from build123d import *

# Parameters (mm, degrees)
SKETCH_1_W          = 280
SKETCH_1_H          = 274
EXTRUDE_1_DEPTH     = 18
SKETCH_2_W          = 520
SKETCH_2_H          = 10
EXTRUDE_2_DEPTH     = 172
CUT_EXTRUDE_1_DEPTH = 466.041933593
CUT_EXTRUDE_2_DEPTH = 466.041933593
SKETCH_5_R          = 11
CUT_EXTRUDE_3_DEPTH = 521.745619281
SKETCH_6_R          = 11
CUT_EXTRUDE_4_DEPTH = 521.745619281
SKETCH_7_R          = 11
CUT_EXTRUDE_5_DEPTH = 521.745619281
SKETCH_8_R          = 11
CUT_EXTRUDE_6_DEPTH = 521.745619281
SKETCH_9_R          = 11
CUT_EXTRUDE_8_DEPTH = 466.041933593


with BuildPart() as part:
    # 草图1 → 拉伸1 (new body)
    with BuildSketch(Plane.XY):
        with Locations((140, 137)):
            Rectangle(SKETCH_1_W, SKETCH_1_H)
    extrude(amount=EXTRUDE_1_DEPTH)

    # 草图2 → 拉伸2 (add)
    with BuildSketch(Plane.XY.offset(18)):
        with Locations((140, 137)):
            Rectangle(SKETCH_2_W, SKETCH_2_H)
    extrude(amount=EXTRUDE_2_DEPTH)

    # 草图3 → 切除-拉伸1 (cut, through all)
    with BuildSketch(Plane.XZ.offset(-132)):
        Polygon((0, 18), (-120, 115), (-120, 18), align=None)
    extrude(amount=-CUT_EXTRUDE_1_DEPTH, mode=Mode.SUBTRACT)

    # 草图4 → 切除-拉伸2 (cut, through all)
    with BuildSketch(Plane.XZ.offset(-132)):
        Polygon((400, 115), (280, 18), (400, 18), align=None)
    extrude(amount=-CUT_EXTRUDE_2_DEPTH, mode=Mode.SUBTRACT)

    # 草图5 → 切除-拉伸3 (cut, through all)
    with BuildSketch(Plane(origin=(0, 0, 0), x_dir=(-1, 0, 0), z_dir=(0, 0, -1))):
        with Locations((-210, 35)):
            Circle(SKETCH_5_R)
    extrude(amount=-CUT_EXTRUDE_3_DEPTH, mode=Mode.SUBTRACT)

    # 草图6 → 切除-拉伸4 (cut, through all)
    with BuildSketch(Plane(origin=(0, 0, 0), x_dir=(-1, 0, 0), z_dir=(0, 0, -1))):
        with Locations((-210, 239)):
            Circle(SKETCH_6_R)
    extrude(amount=-CUT_EXTRUDE_4_DEPTH, mode=Mode.SUBTRACT)

    # 草图7 → 切除-拉伸5 (cut, through all)
    with BuildSketch(Plane(origin=(0, 0, 0), x_dir=(-1, 0, 0), z_dir=(0, 0, -1))):
        with Locations((-70, 35)):
            Circle(SKETCH_7_R)
    extrude(amount=-CUT_EXTRUDE_5_DEPTH, mode=Mode.SUBTRACT)

    # 草图8 → 切除-拉伸6 (cut, through all)
    with BuildSketch(Plane(origin=(0, 0, 0), x_dir=(-1, 0, 0), z_dir=(0, 0, -1))):
        with Locations((-70, 239)):
            Circle(SKETCH_8_R)
    extrude(amount=-CUT_EXTRUDE_6_DEPTH, mode=Mode.SUBTRACT)

    # 草图9 → 切除-拉伸8 (cut, through all)
    with BuildSketch(Plane.XZ.offset(-132)):
        with Locations((140, 80)):
            Circle(SKETCH_9_R)
        with Locations((140, 150)):
            Circle(SKETCH_9_R)
        with Locations((-85.189055636, 158.241096139)):
            Circle(SKETCH_9_R)
        with Locations((-32.636595866, 112)):
            Circle(SKETCH_9_R)
        with Locations((365.189055636, 158.241096139)):
            Circle(SKETCH_9_R)
        with Locations((312.636595866, 112)):
            Circle(SKETCH_9_R)
    extrude(amount=-CUT_EXTRUDE_8_DEPTH, mode=Mode.SUBTRACT)


solid = part.part
For this review, take the finished solid that the model builds, in its own axes (mm). A direction names the side the tool comes from. Coordinates: 2 decimals unless noted, no trailing zeros. Write each loop counter-clockwise with the first axis right and the second up, starting at its lowest first coordinate (ties: lowest second). Pieces come first, ordered by that corner, then holes. Notation, with made-up numbers: (83.5, 65) -> (111.5, 65) arc R25 cw to (111.5, 83) -> close; hole circle Ø5 at (55, -21). An arc over 180 degrees is marked (long way). Write each question's results on one line, items separated by ' | '. Start each with the question number.
1) Consider section A-A (x = 70). Write out the cut boundary in (y, z), plus the area to 3 significant figures.
2) Insertion check: pin 1 (17.5 mm diameter, centred on x = 70, y = 239, fed in from +Z); pin 2 (2 mm diameter, centred on x = 145.5, y = 69.5, fed in from +Z); pin 3 (9 mm diameter, centred on y = 83.5, z = 10.5, fed in from -X); pin 4 (3 mm diameter, centred on x = 303, z = 67, fed in from +Y). Each pin has a flat end and moves straight along its axis. Give the tip position at first contact, or say it passes through.
3) Consider section D-D (y = 177.5). Write out the cut boundary in (x, z).
4) The part is to be moulded in two halves that separate along X. For faces 1 (the face through (400, 137, 152)), 2 (the face through (-59.16, 136.93, 65.82)), 3 (the face through (-74.7, 136.93, 161.55)), 4 (the face through (136, 137, 190)), say which applies: +X half, -X half, draft (parallel to the pull), parting line (faces both ways), or undercut.
5) Consider section B-B (y = 35). Write out the cut boundary in (x, z).
6) Consider section C-C (z = 106.5). Write out the cut boundary in (x, y).
7) For faces 5 (the face through (-34.069, 136.93, 122.906)), 6 (the face through (138, 209, 18)), 7 (the face through (138, 67, 18)), list the 3-axis set-ups (+Z, -Z, +X, -X, +Y, -Y) from which the entire face can be reached by the end or side of a thin tool; tool diameter is ignored.
8) Wall thickness on L1, parallel to Z at x = 140, y = 137; L2, parallel to X at y = 90, z = 16.5; L3, parallel to Z at x = 82, y = 118: over which ranges is each line inside the solid? List them lowest first. Write a range as [from, to].
Geometry says:
1) outline: (0, 0) -> (24, 0) -> (24, 18) -> (0, 18) -> close; (46, 0) -> (228, 0) -> (228, 18) -> (142, 18) -> (142, 190) -> (132, 190) -> (132, 18) -> (46, 18) -> close; (250, 0) -> (274, 0) -> (274, 18) -> (250, 18) -> close | area: 5,860 mm^2
2) pin 1: through | pin 2: z = 18 | pin 3: x = 0 | pin 4: y = 142
3) outline: (0, 0) -> (280, 0) -> (280, 18) -> (0, 18) -> close
4) face 1: +X half | face 2: -X half | face 3: undercut | face 4: draft
5) outline: (0, 0) -> (59, 0) -> (59, 18) -> (0, 18) -> close; (81, 0) -> (199, 0) -> (199, 18) -> (81, 18) -> close; (221, 0) -> (280, 0) -> (280, 18) -> (221, 18) -> close
6) outline: (-109.48, 132) -> (-42.16, 132) -> (-42.16, 142) -> (-109.48, 142) -> close; (-23.11, 132) -> (303.11, 132) -> (303.11, 142) -> (-23.11, 142) -> close; (322.16, 132) -> (389.48, 132) -> (389.48, 142) -> (322.16, 142) -> close
7) face 5: +Y, -Y | face 6: +Z, +X, -X, +Y | face 7: +Z, +X, -X, -Y
8) L1: [0, 69], [91, 139], [161, 190] | L2: [0, 280] | L3: [0, 18]
